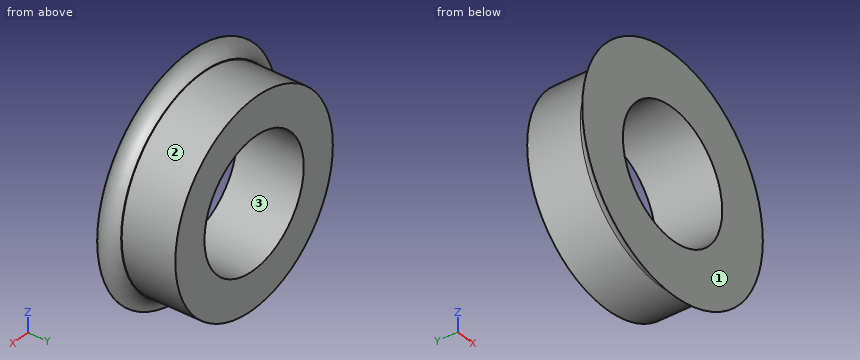
```python
from build123d import *

# Parameters (mm, degrees)
SKETCH_1_R      = 3.925
SKETCH_1_R_2    = 2.475
EXTRUDE_1_DEPTH = 2.57
SKETCH_2_R      = 4.5
SKETCH_2_R_2    = 3.925
EXTRUDE_2_DEPTH = 0.5


with BuildPart() as part:
    # Эскиз1 → Бобышка-Вытянуть1 (new body)
    with BuildSketch(Plane(origin=(0, 0, 0), x_dir=(1, 0, 0), z_dir=(0, 1, 0))):
        Circle(SKETCH_1_R)
        Circle(SKETCH_1_R_2, mode=Mode.SUBTRACT)
    extrude(amount=EXTRUDE_1_DEPTH)

    # Эскиз2 → Бобышка-Вытянуть2 (add)
    with BuildSketch(Plane.XZ):
        Circle(SKETCH_2_R)
        Circle(SKETCH_2_R_2, mode=Mode.SUBTRACT)
    extrude(amount=-EXTRUDE_2_DEPTH)

    # Эскиз3 → Вырез-Повернуть1 (revolve, cut)
    with BuildSketch(Plane.XY):
        with BuildLine():
            Line((-4.5, 0.001444425), (-4.5, 0.5))
            Line((-4.5, 0.5), (-3.95, 0.5))
            ThreePointArc((-3.95, 0.5), (-4.138643926, 0.15545532), (-4.5, 0.001444425))
        make_face()
    revolve(axis=Axis((0, 0, 0), (0, 1, 0)), mode=Mode.SUBTRACT)


solid = part.part
```
Read the model definition and answer for the solid it produces. Units are mm, in the model's axes. Face numbers are marked on the shaded views. Give positions to 0.01 mm unless a question says otherwise; leave off trailing zeros. Write each loop counter-clockwise with the first axis right and the second up, starting at its lowest first coordinate (ties: lowest second). Pieces come first, ordered by that corner, then holes. Notation, with made-up numbers: (24, -27.75) -> (60, -27.75) arc R21 ccw to (60, -15.75) -> close; hole circle Ø1 at (-9, -31). An arc over 180 degrees is marked (long way). Answer in a Markdown table with one row per item.
1) Section C-C on y = 1.2 is taken. Give the vertices of the cut face in (x, z) (3 decimals), plus the area to 3 significant figures.
Results list:
| item | result |
|---|---|
| outline | circle Ø7.85 at (0, 0); hole circle Ø4.95 at (0, 0) |
| area | 29.2 mm^2 |
2) Determine the mould class of the marked faces 1, 2 and 3 for opening direction Z: released by +Z, released by -Z, zero draft, split by the parting line, or undercut.
Results list:
| item | result |
|---|---|
| face 1 | zero draft |
| face 2 | split by the parting line |
| face 3 | undercut |
3) Straight lines are drawn through the part: line 1 (Z direction, x = 0, y = 1.1) (3 decimals); line 2 (X direction, y = 1.3, z = 1.75). For each, find the intervals that lie inside material, in ascending order. Write a range as [from, to].
Results list:
| item | result |
|---|---|
| line 1 | [-3.925, -2.475], [2.475, 3.925] |
| line 2 | [-3.51, -1.75], [1.75, 3.51] |
